Can you work these out from the model? Positions are in its coordinate system, mm. A direction names the side the tool comes from. Coordinates: 2 decimals unless noted, no trailing zeros. Write item = value, one per line.
```python
from build123d import *

# Parameters (mm, degrees)
FILLET1_R     = 0.396875
CHAMFER1_SIZE = 0.127


with BuildPart() as part:
    # Sketch1 → Revolve1 (revolve)
    with BuildSketch(Plane.XY):
        Polygon((2.38125, 0), (4.7625, 0), (4.7625, 1.190625), (3.175, 1.190625), (3.175, 5.159375), (2.38125, 5.159375), align=None)
    revolve(axis=Axis((0, 1.896667818, 0), (0, -1, 0)))

    # Fillet1
    fillet1_edges = [part.edges().sort_by_distance(p)[0] for p in [
        (-3.175, 1.190625, 0),
        (-4.7625, 1.190625, 0),
        (-4.7625, 0, 0),
    ]]
    fillet(fillet1_edges, radius=FILLET1_R)

    # Chamfer1
    chamfer1_edges = [part.edges().sort_by_distance(p)[0] for p in [
        (-2.38125, 5.159375, 0),
        (-3.175, 5.159375, 0),
        (-2.38125, 0, 0),
    ]]
    chamfer(chamfer1_edges, length=CHAMFER1_SIZE)


solid = part.part
```
Item 1: If we mould it in two halves opening along Z, with no side actions, what happens to faces 1 (the cylindrical face through (-3.78, 0.6, -2.9)), 2 (the flat face through (-2, 5.159, -2)), 3 (the cylindrical face through (-1.89, 2.55, -1.45))? For each: pulls with the +Z half, pulls with the -Z half, needs draft (parallel to the pull), parting line crosses it, or undercut.
A:
face_1 = parting line crosses it
face_2 = needs draft
face_3 = undercut
Item 2: If I drill on probe 1 along Z at (x, y) = (0, 3.45) (3 decimals); probe 2 along X at (y, z) = (4.45, -0.5); probe 3 along Y at (x, z) = (-3.75, 2.25), over which ranges is the centre line in solid material (lowest first)?
A:
probe_1 = -3.175 to -2.381, 2.381 to 3.175
probe_2 = -3.14 to -2.33, 2.33 to 3.14
probe_3 = 0 to 1.19
Item 3: For faces 4 (the flat face through (-4, 1.191, 0)), 5 (the flat face through (-2, 0, -2)), which set-ups out of +Z, -Z, +X, -X, +Y, -Y let a thin tool reach every point of the face, with its end or its side?
A:
face_4 = +Y
face_5 = +Z, -Z, +X, -X, -Y
Item 4: I'm going to push flat-ended pins straight in: P1, Ø2, axis at x = -3.5, z = 2.5, coming from the -Y side; P2, Ø2, axis at x = -3.5, y = 1, coming from the -Z side; P3, Ø2, axis at x = 0, y = 3.5, coming from the -Z side (3 decimals). Where does each tip first touch, or does it pass through?
A:
P1 = 0
P2 = -4.04
P3 = -3.175
